Can you work these out from the model? Positions are in its coordinate system, mm. A direction names the side the tool comes from. Coordinates: 2 decimals unless noted, no trailing zeros. Order: outer loops, then holes, each group sorted by start corner. A loop starts at its lowest first (then second) coordinate and runs counter-clockwise, first axis right, second up. Notation, with made-up numbers: (81, -22) - (135, -22) arc R20 ccw to (135, -18) - close; hole circle Ø6 at (68.25, 9). An arc over 180 degrees is marked (long way). Return JSON: item names as keys, results as strings. Group by question number.
1) For pin 1 Ø4 at (x, z) = (-208, 7) entering from -Y; pin 2 Ø5 at (y, z) = (-56, 9.5) entering from -X; pin 3 Ø10 at (x, y) = (81.5, -86.5) entering from -Z, each with a flat end and sliding along its axis, tell me the tip position at first contact or that it passes through.
2) If we mould it in two halves opening along X, with no side actions, what happens to faces 6 (the face through (-1, -96, 30)), 7 (the face through (321.281, -48.437, 14.832)), 8 (the face through (-320.742, -48.437, 14.832)), 9 (the face through (148.43, -97.52, 14.83))? For each: pulls with the +X half, pulls with the -X half, needs draft (parallel to the pull), parting line crosses it, or undercut.
3) If I drill on line 1 along Z through (x, y) = (0, -100.75); line 2 along Y through (x, z) = (7.5, 10); line 3 along Y through (x, z) = (203, 27), over which ranges is the centre line in solid material (lowest first)?
4) Imagine slicing it at A-A (z = 15). Write out the boundary of the cut face in (x, y), and give its area (3 significant figures).
5) Which directions (+Z, -Z, +X, -X, +Y, -Y) give clear straight access to the entire face, cutting with the end or side of a thin tool? Please do faces 1 (the face through (321.372, -62.931, 29.145)), 2 (the face through (-143.821, -98.013, 14.832)), 3 (the face through (-142.04, -83.12, 14.83)), 4 (the face through (-320.96, -49.31, 0.86)), 5 (the face through (-320.95, -49.27, 29.1)).
Autodesk Inventor part; units mm, degrees
ref_plane "YZ Plane" through (0, 0, 0) normal (1, 0, 0) x (0, 1, 0)
ref_plane "XZ Plane" through (0, 0, 0) normal (0, 1, 0) x (-1, 0, 0)
ref_plane "XY Plane" through (0, 0, 0) normal (0, 0, 1) x (1, 0, 0)
sketch "Sketch1" plane through (0, 0, 0) normal (0, 0, 1) x (1, 0, 0)
  arc A0 (0.2695, -91.5776) -> (286.8271, -56.8995) centre (0.2695, 1109.728) ccw
  arc A1 (0.2695, -106.5776) -> (290.4052, -71.4665) centre (0.2695, 1109.728) ccw
  line L0 (0.2695, -106.5776) -> (0.2695, -82.8765)
  line L1 (0, 0) -> (363.543, 0)
  line L2 (286.8271, -56.8995) -> (363.543, -38.0559)
  line L3 (290.4052, -71.4665) -> (353.1517, -56.0541)
  line L4 (363.543, -38.0559) -> (353.1517, -56.0541)
  arc A2 (-286.2882, -56.8995) -> (0.2695, -91.5776) centre (0.2695, 1109.728) ccw
  arc A3 (-289.8663, -71.4665) -> (0.2695, -106.5776) centre (0.2695, 1109.728) ccw
  line L5 (-286.2882, -56.8995) -> (-363.0041, -38.0559)
  line L6 (-289.8663, -71.4665) -> (-352.6128, -56.0541)
  line L7 (-363.0041, -38.0559) -> (-352.6128, -56.0541)
  point P0 (254.9341, -79.6185)
  dimension "d0" = 15
  dimension "d9" = 363.543
extrude "Extrusion1" add sketch "Sketch1" along normal blind 30
sketch "Sketch2" plane through (0, 0, 0) normal (0, 1, 0) x (-1, 0, 0)
  line L0 (0, 0) -> (0, 15)
  circle A0 centre (0, 15) radius 5
  dimension "d5" = 15
  dimension "d6" = 10
extrude "Extrusion2" cut sketch "Sketch2" against normal blind 300
fillet "Fillet2" radius 3 20 edges at (-363.0041, -38.0559, 15) (-357.8084, -47.055, 0) (-357.8084, -47.055, 30) (-352.6128, -56.0541, 15) (146.3957, -97.7679, 30) (321.7784, -63.7603, 30) (-321.2395, -63.7603, 30) (146.3957, -97.7679, 0) (321.7784, -63.7603, 0) (-321.2395, -63.7603, 0) (-144.0547, -82.8765, 30) (325.1851, -47.4777, 30) (-324.6461, -47.4777, 30) (358.3473, -47.055, 30) (363.543, -38.0559, 15) (144.5936, -82.8765, 0) (-324.6461, -47.4777, 0) (325.1851, -47.4777, 0) (358.3473, -47.055, 0) (353.1517, -56.0541, 15)
properties part number "leaf 33" material "Steel, Carbon"
Calculated:
{
 "1": {"pin 1": "y = -88.96", "pin 2": "x = -354.09", "pin 3": "z = 0.02"},
 "2": {"face 6": "needs draft", "face 7": "undercut", "face 8": "undercut", "face 9": "pulls with the +X half"},
 "3": {"line 1": "0 to 10, 20 to 30", "line 2": "-106.56 to -91.56", "line 3": "-89.56 to -74.35"},
 "4": {"outline": "(-359.49, -44.15) - (-353.25, -54.95) arc R3 ccw to (-351.37, -56.36) - (-289.87, -71.47) arc R1216.31 ccw to (-5, -106.57) - (-5, -91.57) arc R1201.31 cw to (-286.29, -56.9) - (-356.17, -39.73) arc R3 ccw to start; (5, -106.57) arc R1216.3 ccw to (290.41, -71.47) - (351.91, -56.36) arc R3 ccw to (353.79, -54.95) - (360.03, -44.15) arc R3 ccw to (356.71, -39.73) - (286.83, -56.9) arc R1201.3 cw to (5, -91.57) - close", "area": "10,700 mm2"},
 "5": {"face 1": "+Z, +X, -Y", "face 2": "+Z, -Z, -X, -Y", "face 3": "+Z, -Z, +Y", "face 4": "-Z, +Y", "face 5": "+Z, +Y"}
}
